Geometry: final body of the model. Coordinates: model frame, mm. Face numbers are marked on the shaded views. A direction names the side the tool comes from. Give positions to 0.01 mm unless a question says otherwise; leave off trailing zeros. Write each loop counter-clockwise with the first axis right and the second up, starting at its lowest first coordinate (ties: lowest second). Pieces come first, ordered by that corner, then holes. Notation, with made-up numbers: (-14.75, 58) -> (0.25, 58) arc R18 cw to (0.25, 75) -> close; hole circle Ø8 at (8, -30). An arc over 180 degrees is marked (long way). Answer as a JSON object with one key per item and string values. Group by question number.
(1) Set-up query: the marked faces 5, 6, 7 and 8. Return all of +Z, -Z, +X, -X, +Y, -Y with unobstructed straight access to the full face (end or side cutting, diameter ignored); none if empty.
(2) Section query D-D on z = -14.5. Output: boundary loops of the cut face in (x, y), plus the area to 3 significant figures.
(3) Section query C-C on x = 0. Output: boundary loops of the cut face in (y, z), plus the area to 3 significant figures.
(4) Section query A-A on z = 0. Output: boundary loops of the cut face in (x, y), plus the area to 3 significant figures.
(5) Material intervals for probe 1 along Y at (x, z) = (7.5, -46); probe 2 along X at (y, z) = (21, -21.5); probe 3 along X at (y, z) = (46, -20), sorted ascending.
(6) Section query B-B on x = -26.5. Output: boundary loops of the cut face in (y, z).
(7) Contact query for flat-ended pins moving along their axis: pin 1 Ø6 at (y, z) = (53, -5) entering from -X; pin 2 Ø11.5 at (y, z) = (16, -13.5) entering from -X; pin 3 Ø6.5 at (x, z) = (-43, -3.5) entering from -Y; pin 4 Ø7.5 at (y, z) = (12.7, 0) entering from -X. Output: stop coordinate, or through.
(8) Draft query along Y for the marked faces 1, 2, 3 and 4. Return one class per face: +Y half, -Y half, draft (parallel to the pull), parting line (faces both ways), or undercut.
from build123d import *

# Parameters (mm, degrees)
F2_W     = 25.4
F2_H     = 38.1
F3_DEPTH = 73.406
F4_W     = 50.8549439785
F4_H     = 94.5440666826
F4_W_2   = 38.6421700465
F4_H_2   = 83.6342661441
F5_DEPTH = 49.022
F6_R     = 6.35
F7_DEPTH = 140.462


with BuildPart() as f1:
    # F0 (on Top) → F1 (revolve)
    with BuildSketch(Plane.XY):
        Polygon((0, 76.2), (0, 0), (50.8, 0), (50.8, 57.15), (44.45, 57.15), (44.45, 63.5), (50.8, 63.5), (50.8, 76.2), align=None)
    revolve(axis=Axis((0, 40.4900377447, 0), (0, 1, 0)))

    # F2 (on Top) → F3 (cut, symmetric)
    with BuildSketch(Plane.XY):
        with Locations((0, 19.05)):
            Rectangle(F2_W, F2_H)
    extrude(amount=F3_DEPTH, both=True, mode=Mode.SUBTRACT)

    # F4 (on face) → F5 (cut)
    with BuildSketch(Plane.XZ):
        with Locations((-63.5274719893, 9.0622203734)):
            Rectangle(F4_W, F4_H)
        with Locations((57.4210850232, -1.1638980359)):
            Rectangle(F4_W_2, F4_H_2)
    extrude(amount=-F5_DEPTH, mode=Mode.SUBTRACT)

    # F6 (on face) → F7 (cut)
    with BuildSketch(Plane(origin=(-38.1, 0, 0), x_dir=(0, -1, 0), z_dir=(-1, 0, 0))):
        with Locations((-12.7, 0)):
            Circle(F6_R)
    extrude(amount=-F7_DEPTH, mode=Mode.SUBTRACT)


solid = f1.part
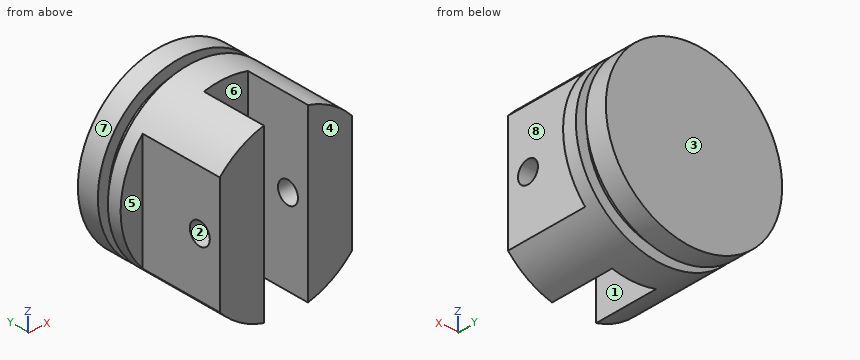
Answer list:
{
 "1": {"face 5": "+Z, -Z, -X, -Y", "face 6": "+Z, -Z, -Y", "face 7": "+Y, -Y", "face 8": "+Z, -Z, +X, -Y"},
 "2": {"outline": "(-48.69, 49.02) -> (-38.1, 49.02) -> (-38.1, 0) -> (-12.7, 0) -> (-12.7, 38.1) -> (12.7, 38.1) -> (12.7, 0) -> (38.1, 0) -> (38.1, 49.02) -> (48.69, 49.02) -> (48.69, 57.15) -> (42.02, 57.15) -> (42.02, 63.5) -> (48.69, 63.5) -> (48.69, 76.2) -> (-48.69, 76.2) -> (-48.69, 63.5) -> (-42.02, 63.5) -> (-42.02, 57.15) -> (-48.69, 57.15) -> close", "area": "5,330 mm2"},
 "3": {"outline": "(38.1, -50.8) -> (57.15, -50.8) -> (57.15, -44.45) -> (63.5, -44.45) -> (63.5, -50.8) -> (76.2, -50.8) -> (76.2, 50.8) -> (63.5, 50.8) -> (63.5, 44.45) -> (57.15, 44.45) -> (57.15, 50.8) -> (38.1, 50.8) -> close", "area": "3,790 mm2"},
 "4": {"outline": "(-50.8, 49.02) -> (-38.1, 49.02) -> (-38.1, 19.05) -> (-12.7, 19.05) -> (-12.7, 38.1) -> (12.7, 38.1) -> (12.7, 19.05) -> (38.1, 19.05) -> (38.1, 49.02) -> (50.8, 49.02) -> (50.8, 57.15) -> (44.45, 57.15) -> (44.45, 63.5) -> (50.8, 63.5) -> (50.8, 76.2) -> (-50.8, 76.2) -> (-50.8, 63.5) -> (-44.45, 63.5) -> (-44.45, 57.15) -> (-50.8, 57.15) -> close; (-38.1, 0) -> (-12.7, 0) -> (-12.7, 6.35) -> (-38.1, 6.35) -> close; (12.7, 0) -> (38.1, 0) -> (38.1, 6.35) -> (12.7, 6.35) -> close", "area": "4,800 mm2"},
 "5": {"probe 1": "38.1 to 57.15, 63.5 to 76.2", "probe 2": "-38.1 to -12.7, 12.7 to 38.1", "probe 3": "-38.1 to 38.1"},
 "6": {"outline": "(0, -43.34) -> (57.15, -43.34) -> (57.15, -35.69) -> (63.5, -35.69) -> (63.5, -43.34) -> (76.2, -43.34) -> (76.2, 43.34) -> (63.5, 43.34) -> (63.5, 35.69) -> (57.15, 35.69) -> (57.15, 43.34) -> (0, 43.34) -> close; hole circle Ø12.7 at (12.7, 0)"},
 "7": {"pin 1": "x = -50.76", "pin 2": "x = -38.1", "pin 3": "y = 49.02", "pin 4": "through"},
 "8": {"face 1": "draft", "face 2": "undercut", "face 3": "+Y half", "face 4": "-Y half"}
}
